Source: CAD feature listing. Evaluate the final solid. Frame: model axes, mm. A direction names the side the tool comes from. Round coordinates to 2 decimals unless told otherwise and drop trailing zeros. Write each loop counter-clockwise with the first axis right and the second up, starting at its lowest first coordinate (ties: lowest second). Pieces come first, ordered by that corner, then holes. Notation, with made-up numbers: M 32,35 L 44,35 A18 cw 44,63 Z; hole C 37.25,-39 d8. An arc over 180 degrees is marked long. Answer in a Markdown table with one row per item. Add a question column.
Item 1: Material intervals for probe 1 along X at (y, z) = (2.25, 0.25) (3 decimals); probe 2 along Y at (x, z) = (9, -0.75); probe 3 along Y at (x, z) = (1.5, 5.5), sorted ascending.
Item 2: Cut plane C-C on z = -1. Give the number of separate pieces and of enclosed holes in the cut face, and give its area (3 significant figures).
Item 3: Set-up query: faces 1 (the face through (-13.804, 0.507, -0.488)), 2 (the face through (17.42, 2.01, -2.5)). Return all of +Z, -Z, +X, -X, +Y, -Y with unobstructed straight access to the full face (end or side cutting, diameter ignored); none if empty.
Item 4: Contact query for flat-ended pins moving along their axis: pin 1 (8 mm diameter, centred on x = 0, z = 8, fed in from -Y); pin 2 (7 mm diameter, centred on x = -16, z = 0, fed in from +Y); pin 3 (0.6 mm diameter, centred on y = 2, z = 0.5, fed in from -X); pin 4 (7 mm diameter, centred on x = -2, z = 1, fed in from +Y). Output: stop coordinate, or through.
Item 5: Cut plane A-A on x = 0. Return loops of the section in (y, z), and give its area (3 significant figures).
Item 6: Cut plane B-B on y = 8. Return loops of the section in (x, z).
Item 7: Mould query, pull axis Z, two halves, no side actions, for faces 3 (the face through (0, 1, 14)), 4 (the face through (3.604, 6.465, 11.446)), 5 (the face through (-14.542, 2.014, -2.478)), 6 (the face through (0, 1, -14)). Classes: released by +Z, released by -Z, zero draft, split by the parting line, or undercut.
from build123d import *

# Parameters (mm, degrees)
SKETCH2_W           = 40
SKETCH2_H           = 28
BOSS_EXTRUDE1_DEPTH = 3
SKETCH3_R           = 12
SKETCH3_R_2         = 11
BOSS_EXTRUDE2_DEPTH = 6
CUT_EXTRUDE1_DEPTH  = 2
FILLET1_R           = 1
FILLET2_R           = 15
SKETCH8_R           = 6.75
CUT_EXTRUDE2_DEPTH  = 0.5
SKETCH9_R           = 2
CUT_EXTRUDE3_DEPTH  = 26.237200627


with BuildPart() as part:
    # Sketch2 → Boss-Extrude1 (new body)
    with BuildSketch(Plane(origin=(0, 0, 0), x_dir=(1, 0, 0), z_dir=(0, 1, 0))):
        Rectangle(SKETCH2_W, SKETCH2_H)
    extrude(amount=BOSS_EXTRUDE1_DEPTH)

    # Sketch3 → Boss-Extrude2 (add)
    with BuildSketch(Plane(origin=(0, 3, 0), x_dir=(1, 0, 0), z_dir=(0, 1, 0))):
        with Locations(Location((0, 0, 0), (0, 0, 270))):
            Circle(SKETCH3_R)
        with Locations(Location((0, 0, 0), (0, 0, 270))):
            Circle(SKETCH3_R_2, mode=Mode.SUBTRACT)
    extrude(amount=BOSS_EXTRUDE2_DEPTH)

    # Sketch4 → Cut-Extrude1 (cut)
    with BuildSketch(Plane(origin=(0, 3, 0), x_dir=(1, 0, 0), z_dir=(0, 1, 0))):
        Polygon((-16, 3.319764048), (-18.875, 1.659882024), (-18.875, -1.659882024), (-16, -3.319764048), (-13.125, -1.659882024), (-13.125, 1.659882024), align=None)
    cut_extrude1 = extrude(amount=-CUT_EXTRUDE1_DEPTH, mode=Mode.SUBTRACT)

    # Sketch6 → M4 Clearance Hole1 (revolve, cut)
    with BuildSketch(Plane(origin=(-16, 1, 0), x_dir=(0, 0, 1), z_dir=(1, 0, 0))):
        Polygon((0, 0), (0, 3.351936393), (2.25, 2), (2.25, 0), align=None)
    m4_clearance_hole1 = revolve(axis=Axis((-16, 7.35, 0), (0, -1, 0)), mode=Mode.SUBTRACT)

    # Mirror1: Cut-Extrude1, M4 Clearance Hole1 across plane
    add(cut_extrude1.mirror(Plane(origin=(0, 0, 0), x_dir=(0, 0, 1), z_dir=(1, 0, 0))), mode=Mode.SUBTRACT)
    add(m4_clearance_hole1.mirror(Plane(origin=(0, 0, 0), x_dir=(0, 0, 1), z_dir=(1, 0, 0))), mode=Mode.SUBTRACT)

    # Fillet1
    fillet1_edges = [part.edges().sort_by_distance(p)[0] for p in [
        (0, 3, -12),
    ]]
    fillet(fillet1_edges, radius=FILLET1_R)

    # Fillet2
    # the kernel refuses this fillet: 15 mm, written as the material it takes off along each edge
    with BuildSketch(Plane(origin=(-20, -37.5, -14), x_dir=(1, 0, 0), z_dir=(0, 1, 0)), Plane(origin=(-20, -37.5, 14), x_dir=(0, 0, -1), z_dir=(0, 1, 0))) as fillet2_piece_1:
        with BuildLine():
            CenterArc((FILLET2_R, -FILLET2_R), FILLET2_R, 90, 90)
            Line((0, -FILLET2_R), (0, 0))
            Line((0, 0), (FILLET2_R, 0))
        make_face()
    extrude(amount=78, mode=Mode.SUBTRACT)
    with BuildSketch(Plane(origin=(20, -37.5, 14), x_dir=(0, 0, -1), z_dir=(0, 1, 0)), Plane(origin=(20, -37.5, -14), x_dir=(-1, 0, 0), z_dir=(0, 1, 0))) as fillet2_piece_2:
        with BuildLine():
            CenterArc((FILLET2_R, FILLET2_R), FILLET2_R, 180, 90)
            Line((0, FILLET2_R), (0, 0))
            Line((0, 0), (FILLET2_R, 0))
        make_face()
    extrude(amount=78, mode=Mode.SUBTRACT)

    # Sketch8 → Cut-Extrude2 (cut)
    with BuildSketch(Plane(origin=(0, 3, 0), x_dir=(1, 0, 0), z_dir=(0, 1, 0))):
        with Locations(Location((0, 0, 0), (0, 0, 270))):
            Circle(SKETCH8_R)
    extrude(amount=-CUT_EXTRUDE2_DEPTH, mode=Mode.SUBTRACT)

    # Sketch9 → Cut-Extrude3 (cut, through all)
    with BuildSketch(Plane(origin=(0, 2.5, 0), x_dir=(1, 0, 0), z_dir=(0, 1, 0))):
        with Locations(Location((0, 0, 0), (0, 0, 270))):
            Circle(SKETCH9_R)
    extrude(amount=-CUT_EXTRUDE3_DEPTH, mode=Mode.SUBTRACT)


solid = part.part
Results below:
| question | item | result |
|---|---|---|
| 1 | probe 1 | -19.948 to -18.875, -13.125 to -1.984, 1.984 to 13.125, 18.875 to 19.948 |
| 1 | probe 2 | 0 to 3 |
| 1 | probe 3 | 0 to 2.5 |
| 2 | separate pieces | 4 |
| 2 | enclosed holes | 0 |
| 2 | area | 85.3 mm2 |
| 3 | face 1 | +Y, -Y |
| 3 | face 2 | +Y |
| 4 | pin 1 | y = 0 |
| 4 | pin 2 | y = 3.13 |
| 4 | pin 3 | x = -19.95 |
| 4 | pin 4 | y = 2.5 |
| 5 | outline | M 0,-14 L 3,-14 L 3,-13 A1 cw 4,-12 L 9,-12 L 9,-11 L 3,-11 L 3,-6.75 L 2.5,-6.75 L 2.5,-2 L 0,-2 Z; M 0,2 L 2.5,2 L 2.5,6.75 L 3,6.75 L 3,11 L 9,11 L 9,12 L 4,12 A1 cw 3,13 L 3,14 L 0,14 Z |
| 5 | area | 79.7 mm2 |
| 6 | outline | C 0,0 d24; hole C 0,0 d22 |
| 7 | face 3 | released by +Z |
| 7 | face 4 | split by the parting line |
| 7 | face 5 | undercut |
| 7 | face 6 | released by -Z |
